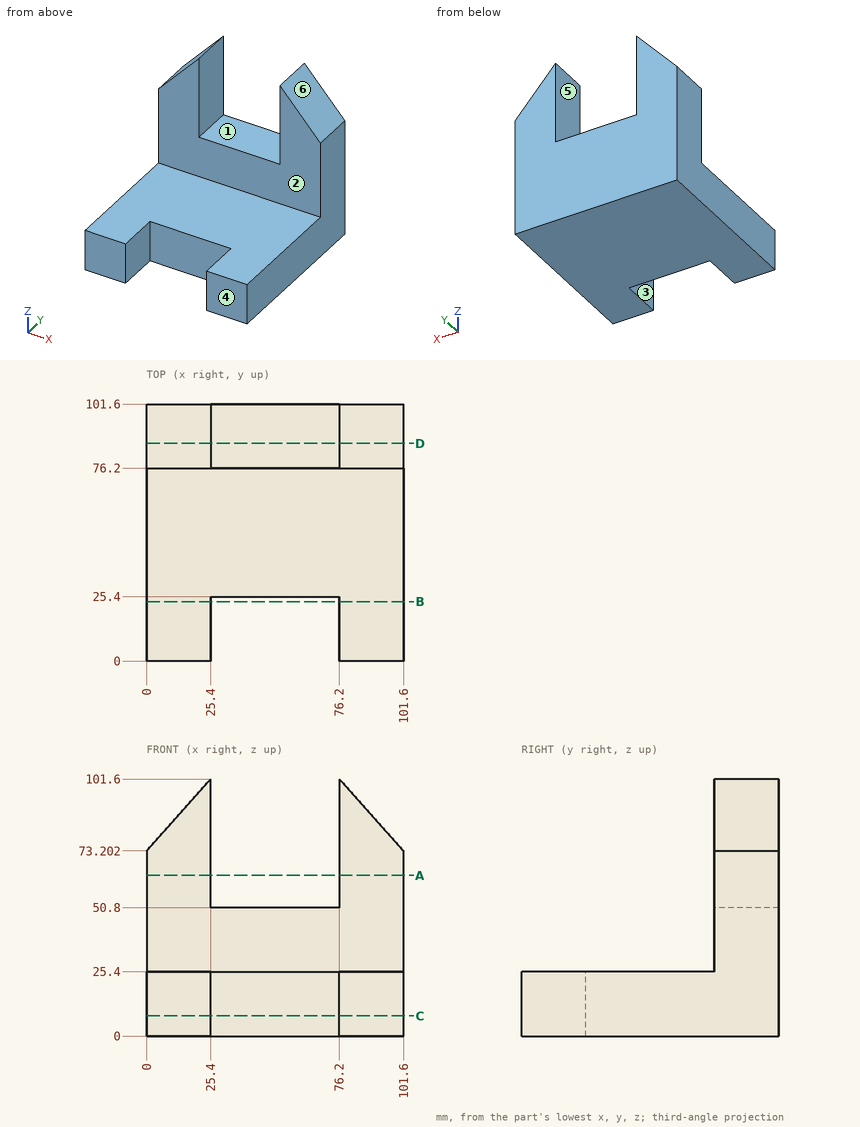
Drawing for the job (mm, zero at the part's lowest x, y, z). A direction names the side the tool comes from. Coordinates: 2 decimals unless noted, no trailing zeros. Loops run counter-clockwise (first coordinate to the right, second up) from the corner with the lowest first, then second, coordinate; pieces in that order, holes last. Notation, with made-up numbers: (79, 77) - (87, 77) arc R23 ccw to (87, 87) - close; hole circle Ø2 at (3.5, 65.25). An arc over 180 degrees is marked (long way). Return JSON: item names as keys, results as strings.
1. Band-saw the part on A-A (z = 63.5). Give the cut face in (x, y).
Result:
{"outline": "(0, 76.2) - (25.4, 76.2) - (25.4, 101.6) - (0, 101.6) - close; (76.2, 76.2) - (101.6, 76.2) - (101.6, 101.6) - (76.2, 101.6) - close"}
2. Band-saw the part on D-D (y = 86). Give the cut face in (x, z), and give its area (3 significant figures).
Result:
{"outline": "(0, 0) - (101.6, 0) - (101.6, 73.2) - (76.2, 101.6) - (76.2, 50.8) - (25.4, 50.8) - (25.4, 101.6) - (0, 73.2) - close", "area": "7,020 mm2"}
3. Drop flat-ended pins along their axis: pin 1 (23 mm diameter, centred on x = 68.5, y = 36, fed in from +Z); pin 2 (8 mm diameter, centred on y = 12, z = 29.5, fed in from -X); pin 3 (12.5 mm diameter, centred on x = 51, y = 88, fed in from +Z); pin 4 (12.5 mm diameter, centred on x = 55.5, z = 17.5, fed in from -Y). Give the stop position or say it passes through.
Result:
{"pin 1": "stops at z = 25.4", "pin 2": "passes through", "pin 3": "stops at z = 50.8", "pin 4": "stops at y = 25.4"}
4. Mould opens along X. For the marked faces 4, 5 and 6 say: released by +X, released by -X, zero draft, split by the parting line, or undercut.
Result:
{"face 4": "zero draft", "face 5": "undercut", "face 6": "released by +X"}
5. 3-axis set-ups, long thin cutter, end or side, ignore diameter. For the marked faces 1, 2 and 3: which of +Z, -Z, +X, -X, +Y, -Y reach the whole face in a straight line?
Result:
{"face 1": "+Z, +Y, -Y", "face 2": "+Z, +X, -X, -Y", "face 3": "+Z, -Z, -Y"}
6. Probe L1, parallel to X at y = 81.5, z = 69; L2, parallel to Y at x = 33.5, z = 40.5; L3, parallel to Y at x = 47.5, z = 24. List the from-to ranges inside material, lowest first. Write a range as from..to.
Result:
{"L1": "x = 0..25.4, 76.2..101.6", "L2": "y = 76.2..101.6", "L3": "y = 25.4..101.6"}
7. Band-saw the part on B-B (y = 23.5). Give the cut face in (x, z).
Result:
{"outline": "(0, 0) - (25.4, 0) - (25.4, 25.4) - (0, 25.4) - close; (76.2, 0) - (101.6, 0) - (101.6, 25.4) - (76.2, 25.4) - close"}
8. Band-saw the part on C-C (z = 8). Give the cut face in (x, y).
Result:
{"outline": "(0, 0) - (25.4, 0) - (25.4, 25.4) - (76.2, 25.4) - (76.2, 0) - (101.6, 0) - (101.6, 101.6) - (0, 101.6) - close"}
